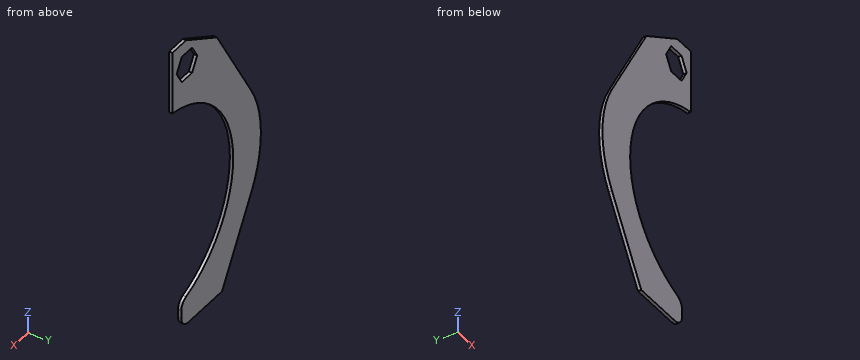
```python
from build123d import *

# Parameters (mm, degrees)
BOSS_EXTRUDE1_DEPTH = 1.5875
CUT_EXTRUDE1_DEPTH  = 1.5875
FILLET1_R           = 5.08
CHAMFER1_SIZE2      = 21.997045256
CHAMFER1_SIZE       = 12.7
FILLET2_R           = 50.8


with BuildPart() as part:
    # Sketch1 → Boss-Extrude1 (new body)
    with BuildSketch(Plane(origin=(0, 0, 0), x_dir=(1, 0, 0), z_dir=(0, 1, 0))):
        with BuildLine():
            Line((-78.442967332, 0), (-39.221483666, -67.933602458))
            Line((-39.221483666, -67.933602458), (-39.221483666, -80.633602458))
            Line((-39.221483666, -80.633602458), (-7.471483666, -80.633602458))
            Line((-7.471483666, -80.633602458), (-7.471483666, -67.933602458))
            Line((-7.471483666, -67.933602458), (-7.471483666, -50.247556476))
            ThreePointArc((-7.471483666, -50.247556476), (-50.696097309, -3.247417072), (-13.821483666, 48.883602458))
            Line((-13.821483666, 48.883602458), (-13.821483666, 61.583602458))
            Line((-13.821483666, 61.583602458), (-42.887657875, 61.583602458))
            Line((-42.887657875, 61.583602458), (-78.442967332, 0))
        make_face()
    extrude(amount=BOSS_EXTRUDE1_DEPTH)

    # Sketch2 → Cut-Extrude1 (cut)
    with BuildSketch(Plane(origin=(0, 1.5875, 0), x_dir=(1, 0, 0), z_dir=(0, 1, 0))):
        Polygon((-10.485751581, -67.933602458), (-14.151925791, -61.583602458), (-21.484274209, -61.583602458), (-25.150448419, -67.933602458), (-21.484274209, -74.283602458), (-14.151925791, -74.283602458), align=None)
    extrude(amount=-CUT_EXTRUDE1_DEPTH, mode=Mode.SUBTRACT)

    # Fillet1
    fillet1_edges = [part.edges().sort_by_distance(p)[0] for p in [
        (-13.821483666, 0.79375, -61.583602458),
        (-13.821483666, 0.79375, -48.883602458),
    ]]
    fillet(fillet1_edges, radius=FILLET1_R)

    # Chamfer1
    chamfer1_edges = [part.edges().sort_by_distance(p)[0] for p in [
        (-39.221483666, 0.79375, 80.633602458),
    ]]
    chamfer1_side = [part.faces().sort_by_distance(p)[0] for p in [
        (-39.221483666, 0.79375, 80.379602458),
    ]]
    chamfer(chamfer1_edges, length=CHAMFER1_SIZE - 0.0001, length2=CHAMFER1_SIZE2 - 0.0001, reference=chamfer1_side[0])  # a hair under: the kernel refuses the full size

    # Fillet2
    fillet2_edges = [part.edges().sort_by_distance(p)[0] for p in [
        (-78.442967332, 0.79375, 0),
    ]]
    fillet(fillet2_edges, radius=FILLET2_R)


solid = part.part
```
Design review of the part built by this model. Coordinates are the model's own, in mm. Coordinates: 2 decimals unless noted, no trailing zeros. Loops run counter-clockwise (first coordinate to the right, second up) from the corner with the lowest first, then second, coordinate; pieces in that order, holes last. Notation, with made-up numbers: (55.5, 61) - (68.5, 61) arc R35 cw to (68.5, 99) - close; hole circle Ø8 at (61.5, 28.25). An arc over 180 degrees is marked (long way). Use CSV: the item, a comma, the result in double quotes. Start each with the question number.
1) Consider section D-D on z = -46. Write out the cut boundary in (x, y).
2) Wall thickness on L1, parallel to Z at x = -20, y = 0.3; L2, parallel to Z at x = -18, y = 1.1; L3, parallel to Z at x = -44.5, y = 1.3: over which ranges is each line inside the solid? List them lowest first. Write a range as from..to.
3) Consider section C-C on x = -23.5. Write out the cut boundary in (y, z), then the cut area to 3 significant figures.
4) Consider section B-B on z = 70. Write out the cut boundary in (x, y).
5) For pin 1 Ø0.5 at (x, y) = (-18, 0.5) entering from +Z, flat-tipped, find the tip position at first contact; note if it passes through.
Geometry says:
1,outline,"(-51.88, 0) - (-21.56, 0) - (-21.56, 1.59) - (-51.88, 1.59) - close"
2,L1,"-61.58..-46.7, 46.7..61.58, 74.28..79.03"
2,L2,"-61.5..-47.5, 47.5..61.58, 74.28..80.19"
2,L3,"-58.79..-24.5, 24.5..58.79"
3,outline,"(0, -61.58) - (1.59, -61.58) - (1.59, -45.04) - (0, -45.04) - close; (0, 45.04) - (1.59, 45.04) - (1.59, 65.07) - (0, 65.07) - close; (0, 70.79) - (1.59, 70.79) - (1.59, 77.01) - (0, 77.01) - close"
3,area,"67.9 mm^2"
4,outline,"(-35.64, 0) - (-23.96, 0) - (-23.96, 1.59) - (-35.64, 1.59) - close; (-11.68, 0) - (-7.47, 0) - (-7.47, 1.59) - (-11.68, 1.59) - close"
5,pin 1,"z = 80.33"
